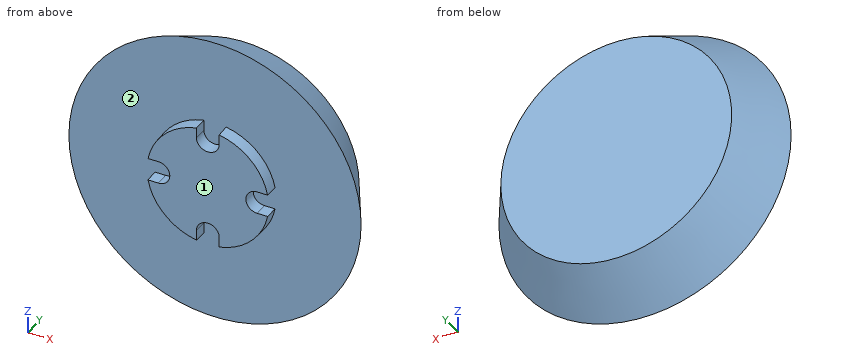
```python
from build123d import *

# Parameters (mm, degrees)
BOSS_EXTRUDE1_DEPTH = 5
BOSS_EXTRUDE1_TAPER = 1


with BuildPart() as part:
    # Sketch2 → Boss-Extrude1 (new body)
    with BuildSketch(Plane(origin=(0, 0, 0), x_dir=(1, 0, 0), z_dir=(0, 1, 0))):
        with BuildLine():
            Line((-4.2, 18.6), (-4.2, 22.61327044))
            ThreePointArc((-4.2, 22.61327044), (-16.263455967, 16.263455967), (-22.61327044, 4.2))
            Line((-22.61327044, 4.2), (-18.6, 4.2))
            ThreePointArc((-18.6, 4.2), (-14.4, 0), (-18.6, -4.2))
            Line((-18.6, -4.2), (-22.61327044, -4.2))
            ThreePointArc((-22.61327044, -4.2), (-16.263455967, -16.263455967), (-4.2, -22.61327044))
            Line((-4.2, -22.61327044), (-4.2, -18.6))
            ThreePointArc((-4.2, -18.6), (0, -14.4), (4.2, -18.6))
            Line((4.2, -18.6), (4.2, -22.61327044))
            ThreePointArc((4.2, -22.61327044), (16.263455967, -16.263455967), (22.61327044, -4.2))
            Line((22.61327044, -4.2), (18.6, -4.2))
            ThreePointArc((18.6, -4.2), (14.4, 0), (18.6, 4.2))
            Line((18.6, 4.2), (22.61327044, 4.2))
            ThreePointArc((22.61327044, 4.2), (16.263455967, 16.263455967), (4.2, 22.61327044))
            Line((4.2, 22.61327044), (4.2, 18.6))
            ThreePointArc((4.2, 18.6), (0, 14.4), (-4.2, 18.6))
        make_face()
    extrude(amount=-BOSS_EXTRUDE1_DEPTH, taper=BOSS_EXTRUDE1_TAPER)

    # Sketch4 → Revolve1 (revolve)
    with BuildSketch(Plane.XY):
        Polygon((0, 0), (55, 0), (43.452994616, 20), (0, 20), align=None)
    revolve(axis=Axis((0, 20, 0), (0, -1, 0)))


solid = part.part
```
Geometry check sheet. Reference: the model listing, model coordinates, mm. Face numbers are marked on the shaded views. A direction names the side the tool comes from. Coordinates: 2 decimals unless noted, no trailing zeros. Order: outer loops, then holes, each group sorted by start corner. A loop starts at its lowest first (then second) coordinate and runs counter-clockwise, first axis right, second up. Notation, with made-up numbers: M 55.5,21 L 91.5,21 A13 cw 91.5,31 Z; hole C -22.5,-19 d10. An arc over 180 degrees is marked long. One line per question, with ' | ' between items. Start each with the question number.
Item 1: Cross-section at A-A on y = 12.5. Enter the section's corners in (x, z), then the cut area to 3 significant figures.
Item 2: Gauge pin test, flat ends, axial feed: pin 1 (1.5 mm diameter, centred on y = 9, z = -9, fed in from +X); pin 2 (2 mm diameter, centred on y = 4.5, z = -19, fed in from -X); pin 3 (1.5 mm diameter, centred on x = -6, y = -2.5, fed in from -Z). Record the tip position at first contact, or that the pin passes through.
Item 3: Material ranges on L1, parallel to Y at x = -35.5, z = 16.5; L2, parallel to X at y = -3.5, z = 1.5; L3, parallel to X at y = -2.5, z = -17.5, recorded low to high. Write a range as [from, to].
Item 4: Set-up check for the marked faces 1 and 2: record each of +Z, -Z, +X, -X, +Y, -Y from which the full face is reachable in a straight line by a thin tool's end or side.
Findings:
1) outline: C 0,0 d95.57 | area: 7,170 mm²
2) pin 1: stops at x = 49.44 | pin 2: stops at x = -49.56 | pin 3: stops at z = -22.35
3) L1: y = [0, 20] | L2: x = [-14.61, 14.61] | L3: x = [-14.86, -4.1], [4.1, 14.86]
4) face 1: +Z, -Z, +X, -X, -Y | face 2: -Y
